For this review, take the finished solid that the model builds, in its own axes (mm). Give positions to 0.01 mm unless a question says otherwise; leave off trailing zeros. Loops run counter-clockwise (first coordinate to the right, second up) from the corner with the lowest first, then second, coordinate; pieces in that order, holes last. Notation, with made-up numbers: (24.5, -30) - (52.5, -30) arc R25 cw to (52.5, 7) - close; hole circle Ø3 at (58, -34.75). An arc over 180 degrees is marked (long way). Answer in a Markdown table with one row per item.
```python
from build123d import *

# Parameters (mm, degrees)
MODEL_R             = 2.5
BOSS_EXTRUDE1_DEPTH = 3


with BuildPart() as part:
    # Model → Boss-Extrude1 (new body, symmetric)
    with BuildSketch(Plane(origin=(0, 0, 0), x_dir=(1, 0, 0), z_dir=(0, 1, 0))):
        with BuildLine():
            Line((-34.997168674, -67.443546623), (-34.999805804, -89.200353377))
            Line((-34.999805804, -89.200353377), (-104.999287788, -89.200353377))
            Line((-104.999287788, -89.200353377), (-105.000194196, 89.200353377))
            Line((-105.000194196, 89.200353377), (104.999740995, 89.200353377))
            Line((104.999740995, 89.200353377), (104.999740995, -89.200353377))
            Line((104.999740995, -89.200353377), (35.000194196, -89.200353377))
            Line((35.000194196, -89.200353377), (35.002831326, -67.443546623))
            ThreePointArc((35.002831326, -67.443546623), (0.002831326, -32.443546623), (-34.997168674, -67.443546623))
        make_face()
        with Locations((52.000194196, -67.443546623)):
            Circle(MODEL_R, mode=Mode.SUBTRACT)
        with Locations((-51.999805804, -67.443546623)):
            Circle(MODEL_R, mode=Mode.SUBTRACT)
        with Locations((-86.999805804, -67.443546623)):
            Circle(MODEL_R, mode=Mode.SUBTRACT)
        with Locations((87.000194196, -67.443546623)):
            Circle(MODEL_R, mode=Mode.SUBTRACT)
    extrude(amount=BOSS_EXTRUDE1_DEPTH, both=True)


solid = part.part
```
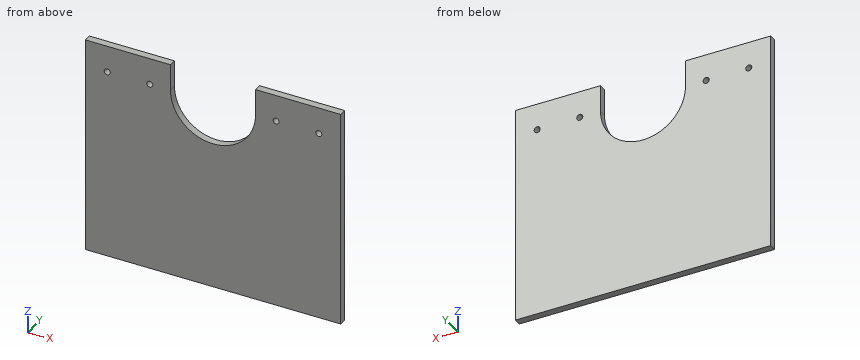
1. We need section A-A, the plane y = -0.65. Give the boundary of the cut face in (x, z).
Values:
| item | result |
|---|---|
| outline | (-105, -89.2) - (105, -89.2) - (105, 89.2) - (35, 89.2) - (35, 67.44) arc R35 cw to (-35, 67.44) - (-35, 89.2) - (-105, 89.2) - close; hole circle Ø5 at (-87, 67.44); hole circle Ø5 at (-52, 67.44); hole circle Ø5 at (52, 67.44); hole circle Ø5 at (87, 67.44) |
2. Wall thickness on line 1 (X direction, y = 1, z = 38); line 2 (X direction, y = 0.3, z = 49); line 3 (Z direction, x = 8, y = -2.6): over which ranges is each line inside the solid? List them lowest first. Write a range as [from, to].
Values:
| item | result |
|---|---|
| line 1 | x = [-105, -18.92], [18.93, 105] |
| line 2 | x = [-105, -29.74], [29.75, 105] |
| line 3 | z = [-89.2, 33.37] |
3. We need section C-C, the plane x = -18. Give the boundary of the cut face in (y, z).
Values:
| item | result |
|---|---|
| outline | (-3, -89.2) - (3, -89.2) - (3, 37.43) - (-3, 37.43) - close |
4. Clearance check with flat-ended pins moving along their axes: pin 1 (1.5 mm diameter, centred on x = -28.5, y = 1, fed in from +Z); pin 2 (1 mm diameter, centred on x = -24.5, y = -1.5, fed in from +Z). State where each tip first meets the part, or that it passes through.
Values:
| item | result |
|---|---|
| pin 1 | stops at z = 48.23 |
| pin 2 | stops at z = 42.95 |
5. We need section B-B, the plane z = 57. Give the boundary of the cut face in (x, y).
Values:
| item | result |
|---|---|
| outline | (-105, -3) - (-33.4, -3) - (-33.4, 3) - (-105, 3) - close; (33.41, -3) - (105, -3) - (105, 3) - (33.41, 3) - close |
6. We need section D-D, the plane x = 27. Give the boundary of the cut face in (y, z), and give its area (3 significant figures).
Values:
| item | result |
|---|---|
| outline | (-3, -89.2) - (3, -89.2) - (3, 45.17) - (-3, 45.17) - close |
| area | 806 mm^2 |
